CAD build for the part. Positions are in the model's coordinates, mm. A direction names the side the tool comes from. Round coordinates to 2 decimals unless told otherwise and drop trailing zeros. Loops run counter-clockwise (first coordinate to the right, second up) from the corner with the lowest first, then second, coordinate; pieces in that order, holes last.
Autodesk Inventor part; units mm, degrees
ref_plane "YZ Plane" through (0, 0, 0) normal (1, 0, 0) x (0, 1, 0)
ref_plane "XZ Plane" through (0, 0, 0) normal (0, 1, 0) x (-1, 0, 0)
ref_plane "XY Plane" through (0, 0, 0) normal (0, 0, 1) x (1, 0, 0)
sketch "Sketch1" plane through (0, 0, 0) normal (0, 1, 0) x (-1, 0, 0)
  line L0 (0, 0) -> (25.4, 0)
  line L1 (25.4, 0) -> (25.4, -50.8)
  line L2 (25.4, -50.8) -> (0, -50.8)
  line L3 (0, -50.8) -> (0, 0)
  line L4 (3.175, -47.625) -> (22.225, -47.625)
  line L5 (22.225, -47.625) -> (22.225, -3.175)
  line L6 (22.225, -3.175) -> (3.175, -3.175)
  line L7 (3.175, -3.175) -> (3.175, -47.625)
  dimension "d0" = 50.8
  dimension "d1" = 25.4
  dimension "d2" = 3.175
extrude "Extrusion1" add sketch "Sketch1" along normal blind 50.8
sketch "Sketch2" plane through (0, 50.8, 0) normal (0, 1, 0) x (1, 0, 0)
  line L0 (-3.175, 47.625) -> (-3.175, 3.175)
  line L1 (-3.175, 3.175) -> (-22.225, 3.175)
  line L2 (-22.225, 3.175) -> (-22.225, 47.625)
  line L3 (-22.225, 47.625) -> (-3.175, 47.625)
  line L4 (-25.4, 0) -> (0, 0)
  line L5 (0, 0) -> (0, 50.8)
  line L6 (0, 50.8) -> (-25.4, 50.8)
  line L7 (-25.4, 50.8) -> (-25.4, 0)
extrude "Extrusion2" add sketch "Sketch2" along normal blind 12.7
sketch "Sketch3" plane through (0, 63.5, 0) normal (0, 1, 0) x (1, 0, 0)
  line L0 (-3.175, 3.175) -> (-22.225, 3.175)
  line L1 (-22.225, 3.175) -> (-22.225, 47.625)
  line L2 (-22.225, 47.625) -> (-3.175, 47.625)
  line L3 (-3.175, 47.625) -> (-3.175, 3.175)
  line L4 (-25.4, 0) -> (0, 0)
  line L5 (0, 0) -> (0, 50.8)
  line L6 (0, 50.8) -> (-25.4, 50.8)
  line L7 (-25.4, 50.8) -> (-25.4, 0)
extrude "Extrusion3" add sketch "Sketch3" along normal blind 6.35
sketch "Sketch4" plane through (-25.4, 0, 0) normal (0, 0, 1) x (1, 0, 0)
  circle A0 centre (12.7, 12.7) radius 2.0701
  line L0 (25.4, 0) -> (0, 0)
  line L1 (25.4, 0) -> (25.4, 69.85)
  dimension "d9" = 4.1402
  dimension "d10" = 12.7
  dimension "d11" = 12.7
extrude "Extrusion4" cut sketch "Sketch4" against normal blind 25.4
properties part number "2x1 2in Alluminum Block.ver1-1111-2019"
Item 1: Cut at C-C, the plane z = -43.5. Give the cut face in (x, y) (3 decimals), plus the area to 3 significant figures.
Answers follow:
outline: (-25.4, 0) - (-22.225, 0) - (-22.225, 69.85) - (-25.4, 69.85) - close; (-3.175, 0) - (0, 0) - (0, 69.85) - (-3.175, 69.85) - close
area: 444 mm2
Item 2: Probe line 1 (X direction, y = 40, z = -38) (3 decimals); line 2 (Z direction, x = -14.5, y = 23.5) (3 decimals); line 3 (Y direction, x = -12.7, z = -1.4). List the from-to ranges inside material, lowest first.
Answers follow:
line 1: x = -25.4 to -22.225, -3.175 to 0
line 2: z = -50.8 to -47.625, -3.175 to 0
line 3: y = 0 to 10.63, 14.77 to 69.85
Item 3: Flat gauge pin, fed straight in: P1, Ø5, axis at y = 48.5, z = -23.5, coming from the +X side. Where does the tip first touch, or does it go through?
Answers follow:
P1: stops at x = 0
Item 4: Cut at D-D, the plane y = 12.7. Give the cut face in (x, z) (3 decimals), plus the area to 3 significant figures.
Answers follow:
outline: (-25.4, -50.8) - (0, -50.8) - (0, 0) - (-10.63, 0) - (-10.63, -3.175) - (-3.175, -3.175) - (-3.175, -47.625) - (-22.225, -47.625) - (-22.225, -3.175) - (-14.77, -3.175) - (-14.77, 0) - (-25.4, 0) - close
area: 430 mm2
Item 5: Cut at A-A, the plane x = -12.7. Give the cut face in (y, z) (3 decimals).
Answers follow:
outline: (0, -50.8) - (69.85, -50.8) - (69.85, -47.625) - (0, -47.625) - close; (0, -3.175) - (10.63, -3.175) - (10.63, 0) - (0, 0) - close; (14.77, -3.175) - (69.85, -3.175) - (69.85, 0) - (14.77, 0) - close
Item 6: Two-plate mould, pull along X, no slides. Class faces 4 (the flat face through (-13, 34, -3.175)), 5 (the flat face through (-2, 0, -27)), 6 (the flat face through (-25.4, 34, -26)), 7 (the flat face through (0, 34, -25)): released by +X, released by -X, zero draft, split by the parting line, or undercut.
Answers follow:
face 4: undercut
face 5: zero draft
face 6: released by -X
face 7: released by +X
Item 7: Cut at B-B, the plane y = 60. Give the cut face in (x, z) (3 decimals), plus the area to 3 significant figures.
Answers follow:
outline: (-25.4, -50.8) - (0, -50.8) - (0, 0) - (-25.4, 0) - close; hole (-22.225, -47.625) - (-3.175, -47.625) - (-3.175, -3.175) - (-22.225, -3.175) - close
area: 444 mm2
Item 8: 3-axis set-ups, long thin cutter, end or side, ignore diameter. For faces 1 (the flat face through (-22.225, 34, -25)), 2 (the flat face through (-23, 69.85, -24)), 3 (the cylindrical face through (-12.969, 14.752, -1.565)): which of +Z, -Z, +X, -X, +Y, -Y reach the whole face in a straight line?
Answers follow:
face 1: +Y, -Y
face 2: +Z, -Z, +X, -X, +Y
face 3: +Z
